Geometry: see drawing. Coordinates: mm, zero at the bounding-box minimum. A direction names the side the tool comes from. Round coordinates to 2 decimals unless told otherwise and drop trailing zeros. Order: outer loops, then holes, each group sorted by start corner. A loop starts at its lowest first (then second) coordinate and runs counter-clockwise, first axis right, second up. Notation, with made-up numbers: (80, 2) -> (137, 2) arc R21 ccw to (137, 26) -> close; hole circle Ø1 at (-15, 58). An arc over 180 degrees is marked (long way). Write item = value, one per line. Start each with the question number.
(1) Ray query, line 1 (Y direction, x = 14.5, z = 20); line 2 (X direction, y = 13.5, z = 24); line 3 (Y direction, x = 11.75, z = 20). Return the intervals inside material, ascending.
(2) Cut plane C-C on z = 22. Return the cut outline in (x, y), then the cut area to 3 significant figures.
(3) Reachability of the marked faces 1, 2 and 3 from +Z, -Z, +X, -X, +Y, -Y: full face, straight path, thin tool, end or side. Return the list, or none.
(4) Contact query for flat-ended pins moving along their axis: pin 1 Ø8 at (y, z) = (39, 20) entering from +X; pin 2 Ø10 at (x, z) = (20.5, 33.5) entering from +Y; pin 3 Ø3 at (x, y) = (12, 34.5) entering from -Z; pin 4 Ø8 at (y, z) = (11, 12.5) entering from +X. Output: stop coordinate, or through.
(5) Cut plane A-A on x = 14. Give the number of separate pieces and of enclosed holes in the cut face, then the cut area to 3 significant figures.
(6) Draft query along Z for the marked faces 4, 5, 6 and 7. Return one class per face: released by +Z, released by -Z, zero draft, split by the parting line, or undercut.
(7) Cut plane B-B on y = 14. Return the cut outline in (x, z).
(8) Cut plane D-D on x = 7.5. Return the cut outline in (y, z).
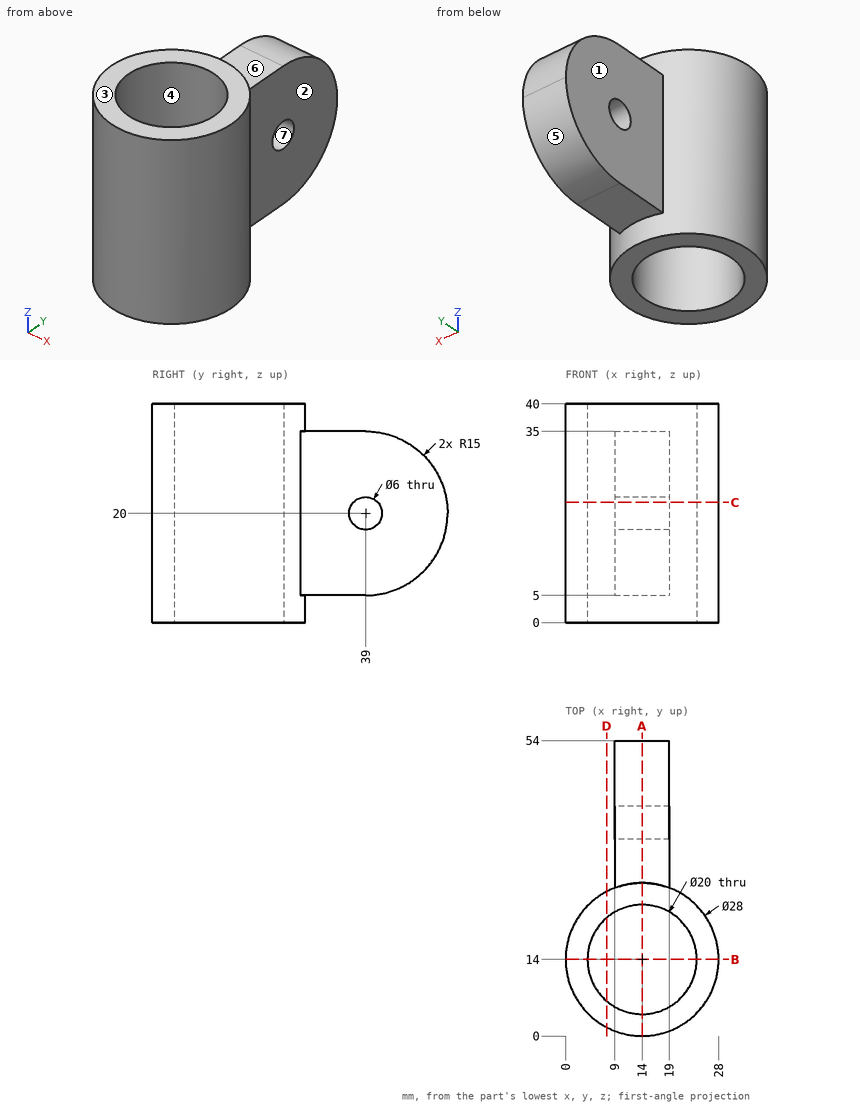
Evaluation:
q1.line_1 = 0.01 to 4.01, 23.99 to 36, 42 to 54
q1.line_2 = 0.01 to 4.01, 23.99 to 27.99
q1.line_3 = 0.18 to 4.26, 23.74 to 36, 42 to 54
q2.outline = (9, 27.08) arc R14 ccw (long way) to (19, 27.08) -> (19, 36.76) -> (9, 36.76) -> close; (9, 41.24) -> (19, 41.24) -> (19, 53.87) -> (9, 53.87) -> close; hole circle Ø20 at (14, 14)
q2.area = 519 mm^2
q3.face_1 = +Z, -Z, -X, +Y
q3.face_2 = +Z, -Z, +X, +Y
q3.face_3 = +Z, +X, -X, +Y, -Y
q4.pin_1 = 19
q4.pin_2 = 51.2
q4.pin_3 = 5
q4.pin_4 = 28
q5.separate_pieces = 2
q5.enclosed_holes = 1
q5.area = 975 mm^2
q6.face_4 = zero draft
q6.face_5 = released by -Z
q6.face_6 = released by +Z
q6.face_7 = undercut
q7.outline = (0, 0) -> (4, 0) -> (4, 40) -> (0, 40) -> close; (24, 0) -> (28, 0) -> (28, 40) -> (24, 40) -> close
q8.outline = (1.6, 0) -> (6.4, 0) -> (6.4, 40) -> (1.6, 40) -> close; (21.6, 0) -> (26.4, 0) -> (26.4, 40) -> (21.6, 40) -> close
